from build123d import *

# Parameters (mm, degrees)
CYLINDER009_R          = 1
CYLINDER009_DEPTH      = 5
CYLINDER010_R          = 1
CYLINDER010_DEPTH      = 5
CYLINDER011_R          = 1
CYLINDER011_DEPTH      = 5
CYLINDER008_R          = 1
CYLINDER008_DEPTH      = 5
CYLINDER007_R          = 8
CYLINDER007_DEPTH      = 1.5
CYLINDER013_R          = 2
CYLINDER013_DEPTH      = 48
BOX001_W               = 20
BOX001_H               = 28
BOX001_DEPTH           = 20
CUT001_PLACEMENT_ANGLE = 180


with BuildPart() as cylinder009:
    # Cylinder009 → Cylinder009 (new body)
    with BuildSketch(Plane(origin=(-7.7, 0, 7.7), x_dir=(1, 0, 0), z_dir=(0, 1, 0))):
        Circle(CYLINDER009_R)
    extrude(amount=CYLINDER009_DEPTH)


with BuildPart() as cylinder010:
    # Cylinder010 → Cylinder010 (new body)
    with BuildSketch(Plane(origin=(7.7, 0, -7.7), x_dir=(1, 0, 0), z_dir=(0, 1, 0))):
        Circle(CYLINDER010_R)
    extrude(amount=CYLINDER010_DEPTH)


with BuildPart() as cylinder011:
    # Cylinder011 → Cylinder011 (new body)
    with BuildSketch(Plane(origin=(7.7, 0, 7.7), x_dir=(1, 0, 0), z_dir=(0, 1, 0))):
        Circle(CYLINDER011_R)
    extrude(amount=CYLINDER011_DEPTH)


with BuildPart() as fusion004:
    # Cylinder008 → Cylinder008 (new body)
    with BuildSketch(Plane(origin=(-7.7, 0, -7.7), x_dir=(1, 0, 0), z_dir=(0, 1, 0))):
        Circle(CYLINDER008_R)
    extrude(amount=CYLINDER008_DEPTH)

    # Fusion004: union Cylinder009, Cylinder010, Cylinder011
    add(cylinder009.part)
    add(cylinder010.part)
    add(cylinder011.part)


with BuildPart() as cylinder007:
    # Cylinder007 → Cylinder007 (new body)
    with BuildSketch(Plane(origin=(0, -1.5, 0), x_dir=(1, 0, 0), z_dir=(0, 1, 0))):
        Circle(CYLINDER007_R)
    extrude(amount=CYLINDER007_DEPTH)


with BuildPart() as cylinder013:
    # Cylinder013 → Cylinder013 (new body)
    with BuildSketch(Plane(origin=(0, -12, 0), x_dir=(1, 0, 0), z_dir=(0, 1, 0))):
        Circle(CYLINDER013_R)
    extrude(amount=CYLINDER013_DEPTH)


with BuildPart() as doubleshaftstepper:
    # Box001 → Box001 (new body)
    with BuildSketch(Plane(origin=(-10, 0, -10), x_dir=(1, 0, 0), z_dir=(0, 0, 1))):
        with Locations((10, 14)):
            Rectangle(BOX001_W, BOX001_H)
    extrude(amount=BOX001_DEPTH)

    # Fusion003: union Cylinder007, Cylinder013
    add(cylinder007.part)
    add(cylinder013.part)

    # Cut001: cut Fusion004
    add(fusion004.part, mode=Mode.SUBTRACT)


with BuildPart() as doubleshaftstepper_1:
    # Cut001 placement: moved
    add(doubleshaftstepper.part.moved(Location((0, 42, 30))).rotate(Axis((0, 42, 30), (0, 0, 1)), CUT001_PLACEMENT_ANGLE))


solid = doubleshaftstepper_1.part
Can you work these out from the model? Positions are in its coordinate system, mm. A direction names the side the tool comes from. Coordinates: 2 decimals unless noted, no trailing zeros. Write each loop counter-clockwise with the first axis right and the second up, starting at its lowest first coordinate (ties: lowest second). Pieces come first, ordered by that corner, then holes.
Q1. Imagine slicing it at B-B, the plane z = 31. List the corners of the cut face in (x, y) for me, plus the area to 3 significant figures.
Results found:
outline: (-10, 14) - (-1.73, 14) - (-1.73, 6) - (1.73, 6) - (1.73, 14) - (10, 14) - (10, 42) - (7.94, 42) - (7.94, 43.5) - (1.73, 43.5) - (1.73, 54) - (-1.73, 54) - (-1.73, 43.5) - (-7.94, 43.5) - (-7.94, 42) - (-10, 42) - close
area: 648 mm2
Q2. Please list where these lines run through material, in increasing order: L1, parallel to X at y = 40.5, z = 22.3; L2, parallel to Z at x = -7.7, y = 40.65; L3, parallel to Y at x = -1, z = 32.
Results found:
L1: x = -10 to -8.7, -6.7 to 6.7, 8.7 to 10
L2: z = 20 to 21.3, 23.3 to 36.7, 38.7 to 40
L3: y = 14 to 43.5
Q3. Imagine slicing it at A-A, the plane x = 0. List the corners of the cut face in (y, z) for me.
Results found:
outline: (6, 28) - (14, 28) - (14, 20) - (42, 20) - (42, 22) - (43.5, 22) - (43.5, 28) - (54, 28) - (54, 32) - (43.5, 32) - (43.5, 38) - (42, 38) - (42, 40) - (14, 40) - (14, 32) - (6, 32) - close
Q4. Which directions (+Z, -Z, +X, -X, +Y, -Y) give clear straight access to the entire face, cutting with the end or side of a thin tool? Please do faces 5 (the face through (10, 28, 30)), 6 (the face through (0, 10, 32)), 7 (the face through (7.24, 39.53, 23.19)).
Results found:
face 5: +Z, -Z, +X, +Y, -Y
face 6: -Y
face 7: +Y
Q5. For P1, Ø6, axis at x = -5, z = 33, coming from the -Y side; P2, Ø1.6, axis at x = 8, z = 38, coming from the +Y side; P3, Ø1, axis at x = 8, z = 22.5, coming from the +Y side, each with a flat end and sliding along its axis, tell me the tip position at first contact or that it passes through.
Results found:
P1: stops at y = 14
P2: stops at y = 42
P3: stops at y = 37
Q6. If we mould it in two halves opening along Z, with no side actions, what happens to faces 1 (the face through (0, 28, 20)), 2 (the face through (8, 37, 22)), 3 (the face through (-8, 37, 38)), 4 (the face through (-2, 43.5, 32))? For each: +Z half, -Z half, draft (parallel to the pull), parting line (faces both ways), or undercut.
Results found:
face 1: -Z half
face 2: undercut
face 3: undercut
face 4: draft
Q7. Imagine slicing it at C-C, the plane z = 25. List the corners of the cut face in (x, y) for me (3 decimals), plus the area to 3 significant figures.
Results found:
outline: (-10, 14) - (10, 14) - (10, 42) - (6.245, 42) - (6.245, 43.5) - (-6.245, 43.5) - (-6.245, 42) - (-10, 42) - close
area: 579 mm2
